Could you check a few things on this model? Use its own coordinates, in mm. Face numbers are marked on the shaded views. A direction names the side the tool comes from. Give positions to 0.01 mm unless a question says otherwise; leave off trailing zeros. Loops run counter-clockwise (first coordinate to the right, second up) from the corner with the lowest first, then second, coordinate; pieces in that order, holes last. Notation, with made-up numbers: M 40,40.5 L 77,40.5 A21 ccw 77,53.5 Z; hole C -29,49 d4. An arc over 180 degrees is marked long. Use CSV: the item, a comma, the result in double quotes.
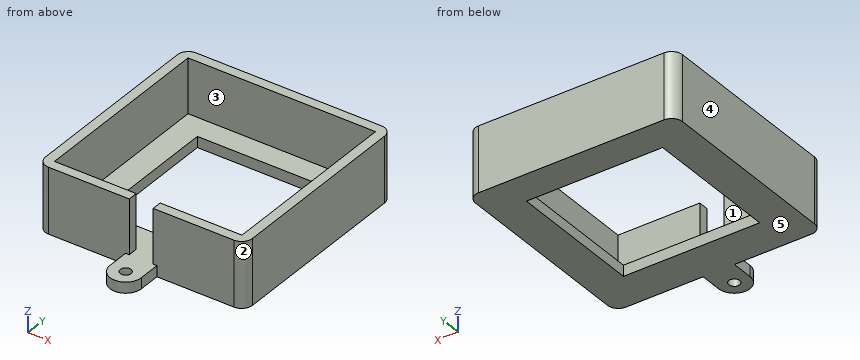
```python
from build123d import *

# Parameters (mm, degrees)
ESQUISSE1_W        = 38
ESQUISSE1_H        = 38
ESQUISSE1_W_2      = 25
ESQUISSE1_H_2      = 25
BOSS_EXTRU_1_DEPTH = 2
BOSS_EXTRU_2_DEPTH = 10
CONG_1_R           = 2
ESQUISSE3_R        = 1
BOSS_EXTRU_3_DEPTH = 2


# Read off the part's stored shape, not the designer's step: Boss.-Extru.2
with BuildPart() as part:
    # Esquisse1 → Boss.-Extru.1 (new body)
    with BuildSketch(Plane.XY):
        with Locations((-5.018947996, 3.742614476)):
            Rectangle(ESQUISSE1_W, ESQUISSE1_H)
        with Locations((-5.018947996, 4.242614476)):
            Rectangle(ESQUISSE1_W_2, ESQUISSE1_H_2, mode=Mode.SUBTRACT)
    extrude(amount=BOSS_EXTRU_1_DEPTH)

    # Boss.-Extru.2 outline → Boss.-Extru.2 (add)
    with BuildSketch(Plane.XY.offset(2)):
        Polygon((-24.018947996, 22.742614476), (-24.018947996, -15.257385524), (-7.218947996, -15.257385524), (-7.218947996, -13.457385524), (-22.218947996, -13.457385524), (-22.218947996, 20.942614476), (12.181052004, 20.942614476), (12.181052004, -13.457385524), (-2.818947996, -13.457385524), (-2.818947996, -15.257385524), (13.981052004, -15.257385524), (13.981052004, 22.742614476), align=None)
    extrude(amount=BOSS_EXTRU_2_DEPTH)

    # Congé1
    cong_1_edges = [part.edges().sort_by_distance(p)[0] for p in [
        (-24.018947996, 22.742614476, 6),
        (13.981052004, 22.742614476, 7),
        (13.981052004, -15.257385524, 7),
        (-24.018947996, -15.257385524, 7),
    ]]
    fillet(cong_1_edges, radius=CONG_1_R)

    # Esquisse3 → Boss.-Extru.3 (add)
    with BuildSketch(Plane(origin=(0, 0, 0), x_dir=(-1, 0, 0), z_dir=(0, 0, -1))):
        with BuildLine():
            Line((2.142498892, -15.257385524), (2.142498892, -19.257385524))
            ThreePointArc((2.142498892, -19.257385524), (5.018947996, -22.133834629), (7.895397101, -19.257385524))
            Line((7.895397101, -19.257385524), (7.895397101, -15.257385524))
            Line((7.895397101, -15.257385524), (2.142498892, -15.257385524))
        make_face()
        with Locations((5.018947996, -19.257385524)):
            Circle(ESQUISSE3_R, mode=Mode.SUBTRACT)
    extrude(amount=-BOSS_EXTRU_3_DEPTH)


solid = part.part
```
1. I'm going to push flat-ended pins straight in: pin 1 Ø1 at (y, z) = (-17, 1) entering from +X; pin 2 Ø2 at (y, z) = (-16.5, 1) entering from -X; pin 3 Ø2.5 at (x, y) = (-5.02, -19.26) entering from -Z; pin 4 Ø5 at (x, z) = (-8.5, 9) entering from -Y. Where does each tip first touch, or does it pass through?
Outcome:
pin 1,"x = -2.14"
pin 2,"x = -7.9"
pin 3,"z = 0"
pin 4,"y = -15.26"
2. Please list where these lines run through material, in increasing order: line 1 (X direction, y = 19, z = 9.5); line 2 (Y direction, x = 12, z = 7.25); line 3 (Y direction, x = -12, z = 0.75).
Outcome:
line 1,"-24.02 to -22.22, 12.18 to 13.98"
line 2,"-15.26 to -13.46, 20.94 to 22.74"
line 3,"-15.26 to -8.26, 16.74 to 22.74"
3. I want a section at D-D, the plane z = 5. List the corners of the cut face in (x, y) for me.
Outcome:
outline,"M -24.02,-13.26 A2 ccw -22.02,-15.26 L -7.22,-15.26 L -7.22,-13.46 L -22.22,-13.46 L -22.22,20.94 L 12.18,20.94 L 12.18,-13.46 L -2.82,-13.46 L -2.82,-15.26 L 11.98,-15.26 A2 ccw 13.98,-13.26 L 13.98,20.74 A2 ccw 11.98,22.74 L -22.02,22.74 A2 ccw -24.02,20.74 Z"
4. I want a section at B-B, the plane y = 11.5. List the corners of the cut face in (x, z) for me.
Outcome:
outline,"M -24.02,0 L -17.52,0 L -17.52,2 L -22.22,2 L -22.22,12 L -24.02,12 Z; M 7.48,0 L 13.98,0 L 13.98,12 L 12.18,12 L 12.18,2 L 7.48,2 Z"
5. If we mould it in two halves opening along X, with no side actions, what happens to the marked faces 3, 4 and 5? For each: +X half, -X half, draft (parallel to the pull), parting line (faces both ways), or undercut.
Outcome:
face 3,"undercut"
face 4,"-X half"
face 5,"draft"
6. Which directions (+Z, -Z, +X, -X, +Y, -Y) give clear straight access to the entire face, cutting with the end or side of a thin tool? Please do the marked faces 1 and 2.
Outcome:
face 1,"+Z"
face 2,"+Z, -Z, +X, -Y"
7. I want a section at A-A, the plane x = -16.5. List the corners of the cut face in (y, z) for me, then the cut area to 3 significant figures.
Outcome:
outline,"M -15.26,0 L -8.26,0 L -8.26,2 L -13.46,2 L -13.46,12 L -15.26,12 Z; M 16.74,0 L 22.74,0 L 22.74,12 L 20.94,12 L 20.94,2 L 16.74,2 Z"
area,"62.0 mm2"
8. I want a section at C-C, the plane z = 1. List the corners of the cut face in (x, y) for me.
Outcome:
outline,"M -24.02,-13.26 A2 ccw -22.02,-15.26 L -7.9,-15.26 L -7.9,-19.26 A2.88 ccw -2.14,-19.26 L -2.14,-15.26 L 11.98,-15.26 A2 ccw 13.98,-13.26 L 13.98,20.74 A2 ccw 11.98,22.74 L -22.02,22.74 A2 ccw -24.02,20.74 Z; hole M -17.52,-8.26 L 7.48,-8.26 L 7.48,16.74 L -17.52,16.74 Z; hole C -5.02,-19.26 d2"
